Geometry check sheet. Reference: drawing and pictorial views, mm from the part's lowest x, y, z. Round coordinates to 2 decimals unless told otherwise and drop trailing zeros. Order: outer loops, then holes, each group sorted by start corner. A loop starts at its lowest first (then second) coordinate and runs counter-clockwise, first axis right, second up.
Q1. Scan lines: probe 1 along Z at (x, y) = (2.54, 0.6); probe 2 along Z at (x, y) = (17.95, 1.1); probe 3 along X at (y, z) = (0.5, 16.62). Record each from-to range of solid material in increasing order.
Q2. Cross-section at B-B on x = 17.95. Record the cut outline in (y, z).
Q3. Cross-section at D-D on y = 0.4. Record the cut outline in (x, z).
Q4. Cross-section at A-A on z = 11.2. Record the cut outline in (x, y).
Q5. Cross-section at C-C on z = 1.38. Record the cut outline in (x, y).
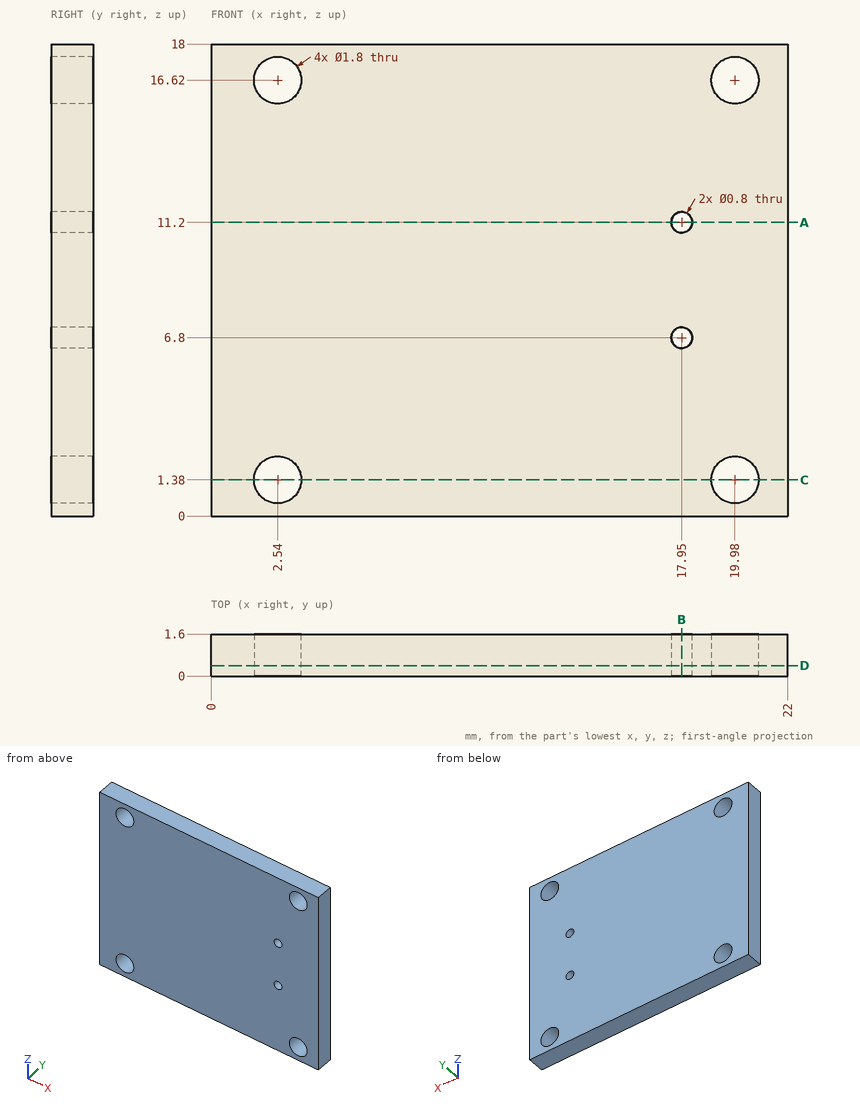
Results found:
1. probe 1: z = 0 to 0.48, 2.28 to 15.72, 17.52 to 18
1. probe 2: z = 0 to 6.4, 7.2 to 10.8, 11.6 to 18
1. probe 3: x = 0 to 1.64, 3.44 to 19.08, 20.88 to 22
2. outline: (0, 0) - (1.6, 0) - (1.6, 6.4) - (0, 6.4) - close; (0, 7.2) - (1.6, 7.2) - (1.6, 10.8) - (0, 10.8) - close; (0, 11.6) - (1.6, 11.6) - (1.6, 18) - (0, 18) - close
3. outline: (0, 0) - (22, 0) - (22, 18) - (0, 18) - close; hole circle Ø1.8 at (2.54, 1.38); hole circle Ø1.8 at (2.54, 16.62); hole circle Ø0.8 at (17.95, 6.8); hole circle Ø0.8 at (17.95, 11.2); hole circle Ø1.8 at (19.98, 1.38); hole circle Ø1.8 at (19.98, 16.62)
4. outline: (0, 0) - (17.55, 0) - (17.55, 1.6) - (0, 1.6) - close; (18.35, 0) - (22, 0) - (22, 1.6) - (18.35, 1.6) - close
5. outline: (0, 0) - (1.64, 0) - (1.64, 1.6) - (0, 1.6) - close; (3.44, 0) - (19.08, 0) - (19.08, 1.6) - (3.44, 1.6) - close; (20.88, 0) - (22, 0) - (22, 1.6) - (20.88, 1.6) - close
